```python
from build123d import *

# Parameters (mm, degrees)
F1_DEPTH = 68.58
F3_DEPTH = 76.201


with BuildPart() as f1:
    # F0 (on Front) → F1 (new body)
    with BuildSketch(Plane.XZ):
        with BuildLine():
            Line((-34.29, 0), (0, 0))
            Line((0, 0), (0, 10.16))
            Line((0, 10.16), (-12.065, 10.16))
            Line((-12.065, 10.16), (-12.065, 40.64))
            Line((-12.065, 40.64), (0, 40.64))
            Line((0, 40.64), (0, 50.8))
            Line((0, 50.8), (-66.04, 50.8))
            ThreePointArc((-66.04, 50.8), (-73.224205, 47.824205), (-76.2, 40.64))
            Line((-76.2, 40.64), (-76.2, 30.48))
            ThreePointArc((-76.2, 30.48), (-73.224205, 23.295795), (-66.04, 20.32))
            Line((-66.04, 20.32), (-43.18, 20.32))
            Line((-43.18, 20.32), (-43.18, 10.16))
            Line((-43.18, 10.16), (-76.2, 10.16))
            Line((-76.2, 10.16), (-76.2, 0))
            Line((-76.2, 0), (-43.18, 0))
            ThreePointArc((-43.18, 0), (-38.019975, 1.407872), (-34.29, 5.241311))
            Line((-34.29, 5.241311), (-34.29, 0))
        make_face()
        with BuildLine():
            Line((-22.225, 10.16), (-33.02, 10.16))
            Line((-33.02, 10.16), (-33.02, 20.32))
            ThreePointArc((-33.02, 20.32), (-35.995795, 27.504205), (-43.18, 30.48))
            Line((-43.18, 30.48), (-66.04, 30.48))
            Line((-66.04, 30.48), (-66.04, 40.64))
            Line((-66.04, 40.64), (-22.225, 40.64))
            Line((-22.225, 40.64), (-22.225, 10.16))
        make_face(mode=Mode.SUBTRACT)
    extrude(amount=F1_DEPTH)

    # F2 (on Right) → F3 (intersect, through all)
    with BuildSketch(Plane.YZ):
        Polygon((-11.43, 0), (0, 40.64), (0, 50.8), (-10.16, 50.8), (-17.78, 15.24), (-25.4, 50.8), (-35.56, 50.8), (-68.58, 50.8), (-68.58, 40.64), (-54.61, 40.64), (-54.61, 0), (-44.45, 0), (-44.45, 40.64), (-35.56, 40.64), (-24.13, 0), align=None)
    extrude(amount=-F3_DEPTH, mode=Mode.INTERSECT)


solid = f1.part
```
Part model, mm, in its own coordinate system. A direction names the side the tool comes from. Round coordinates to 2 decimals unless told otherwise and drop trailing zeros. Loops run counter-clockwise (first coordinate to the right, second up) from the corner with the lowest first, then second, coordinate; pieces in that order, holes last. Notation, with made-up numbers: (-26.5, 52) -> (-22.5, 52) arc R24 ccw to (-22.5, 68) -> close; hole circle Ø2 at (69, -9). An arc over 180 degrees is marked (long way). Use one line per item in the form item = value. Start each with the question number.
Item 1: Band-saw the part on D-D (x = -17.5). List the corners of the cut face in (y, z), plus the area to 3 significant figures.
Item 2: Tool access for faces 1 (the cylindrical face through (-35.917, -25.689, 27.425)), 2 (the cylindrical face through (-73.303, -25.689, 23.375)), 3 (the flat face through (-38, -44.45, 16)): list every direction of +Z, -Z, +X, -X, +Y, -Y with a clear straight run to the whole face (end or side of a thin tool).
Item 3: Band-saw the part on B-B (x = -6). List the corners of the cut face in (y, z).
Item 4: Drill centre lines: line 1 along Z through (x, y) = (-53.5, -47); line 2 along Z through (x, y) = (-63, -8); line 3 along X through (y, z) = (-31.5, 39) (3 decimals). Where is each one in solid material? Low to high.
Item 5: Two-plate mould, pull along X, no slides. Class faces 4 (the flat face through (-59, -49, 10.16)), 5 (the cylindrical face through (-73.145, -45.584, 47.903)), 6 (the cylindrical face through (-35.917, -49.459, 27.425)): released by +X, released by -X, zero draft, split by the parting line, or undercut.
Item 6: Band-saw the part on C-C (z = 42). List the corners of the cut face in (x, y).
Item 7: Band-saw the part on A-A (x = -56). Give the number of separate pieces and of enclosed holes in the cut face, plus the area to 3 significant figures.
Item 8: Drop flat-ended pins along their axis: pin 1 Ø11 at (y, z) = (-48, 23.5) entering from -X; pin 2 Ø5 at (y, z) = (-51, 14) entering from +X (3 decimals); pin 3 Ø12 at (x, z) = (-45, 27) entering from -Y. Give the stop position or say it passes through.
Data:
q1.outline = (-68.58, 40.64) -> (-54.61, 40.64) -> (-54.61, 0) -> (-44.45, 0) -> (-44.45, 40.64) -> (-35.56, 40.64) -> (-24.13, 0) -> (-11.43, 0) -> (0, 40.64) -> (0, 50.8) -> (-10.16, 50.8) -> (-17.78, 15.24) -> (-25.4, 50.8) -> (-68.58, 50.8) -> close
q1.area = 1,820 mm^2
q2.face_1 = +Y, -Y
q2.face_2 = -X, +Y, -Y
q2.face_3 = -Z, +X, -X
q3.outline = (-68.58, 40.64) -> (-23.22, 40.64) -> (-25.4, 50.8) -> (-68.58, 50.8) -> close; (-54.61, 0) -> (-44.45, 0) -> (-44.45, 10.16) -> (-54.61, 10.16) -> close; (-26.99, 10.16) -> (-24.13, 0) -> (-11.43, 0) -> (-8.57, 10.16) -> close; (-12.34, 40.64) -> (0, 40.64) -> (0, 50.8) -> (-10.16, 50.8) -> close
q4.line_1 = 0 to 10.16, 20.32 to 30.48, 40.64 to 50.8
q4.line_2 = 20.32 to 30.48, 40.64 to 50.8
q4.line_3 = -76.2 to -66.04, -22.225 to -12.065
q5.face_4 = zero draft
q5.face_5 = released by -X
q5.face_6 = undercut
q6.outline = (-76.11, -68.58) -> (0, -68.58) -> (0, -23.51) -> (-76.11, -23.51) -> close; (-76.11, -12.05) -> (0, -12.05) -> (0, 0) -> (-76.11, 0) -> close
q7.separate_pieces = 7
q7.enclosed_holes = 0
q7.area = 1,160 mm^2
q8.pin_1 = -76.09
q8.pin_2 = -12.065
q8.pin_3 = -54.61
